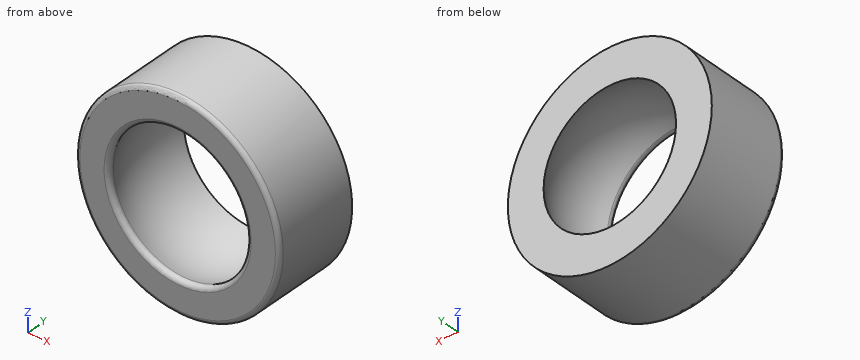
from build123d import *

# Parameters (mm, degrees)
FILLET1_R = 0.3
FILLET2_R = 0.3


with BuildPart() as part:
    # Sketch1 → Revolve1 (revolve)
    with BuildSketch(Plane.XY):
        with BuildLine():
            Line((-4.675256677, 3), (-7.2, 3))
            Line((-7.2, 3), (-7.2, -3))
            Line((-7.2, -3), (-4.675256677, -3))
            ThreePointArc((-4.675256677, -3), (-5.555, 0), (-4.675256677, 3))
        make_face()
    revolve(axis=Axis((0, -3.809768202, 0), (0, 1, 0)))

    # Fillet1
    fillet1_edges = [part.edges().sort_by_distance(p)[0] for p in [
        (4.675256677, -3, 0),
    ]]
    fillet(fillet1_edges, radius=FILLET1_R)

    # Fillet2
    fillet2_edges = [part.edges().sort_by_distance(p)[0] for p in [
        (7.2, -3, 0),
    ]]
    fillet(fillet2_edges, radius=FILLET2_R)


solid = part.part
Read the model definition and answer for the solid it produces. Units are mm, in the model's axes. Round coordinates to 2 decimals unless told otherwise and drop trailing zeros. Loops run counter-clockwise (first coordinate to the right, second up) from the corner with the lowest first, then second, coordinate; pieces in that order, holes last.
Q1. Consider probe 1 along Z at (x, y) = (-3.5, 0); probe 2 along X at (y, z) = (-2.5, 1.75); probe 3 along Z at (x, y) = (-1, -1). Determine where each line is inside the solid, lowest interval first.
Q2. Section B-B on y = -0.75 is taken. Write down the section's boundary in (x, z), and give its area (3 significant figures).
Q3. Section A-A on y = -1.5 is taken. Write down the section's boundary in (x, z).
Q4. Each of these flat-tipped pins is pushed along its axis until it touches: pin 1 (2 mm diameter, centred on x = 2.5, y = 1, fed in from -Z); pin 2 (6 mm diameter, centred on x = 2, z = -1, fed in from -Y). Where does it stop, or does it pass through?
Output:
1. probe 1: z = -6.29 to -4.31, 4.31 to 6.29
1. probe 2: x = -6.98 to -4.64, 4.64 to 6.98
1. probe 3: z = -7.13 to -5.37, 5.37 to 7.13
2. outline: circle Ø14.4 at (0, 0); hole circle Ø11.01 at (0, 0)
2. area: 67.7 mm2
3. outline: circle Ø14.4 at (0, 0); hole circle Ø10.7 at (0, 0)
4. pin 1: stops at z = -7.04
4. pin 2: stops at y = -3
